Can you work these out from the drawing? Everything is in mm from the part's minimum corner. A direction names the side the tool comes from. Coordinates: 2 decimals unless noted, no trailing zeros. Order: outer loops, then holes, each group sorted by start corner. A loop starts at its lowest first (then second) coordinate and runs counter-clockwise, first axis right, second up. Notation, with made-up numbers: (-12.75, 6.5) -> (19.25, 6.5) arc R33 cw to (19.25, 41.5) -> close; hole circle Ø2 at (-36.75, -35). An arc over 180 degrees is marked (long way). Write item = value, one per line. Start each with the question number.
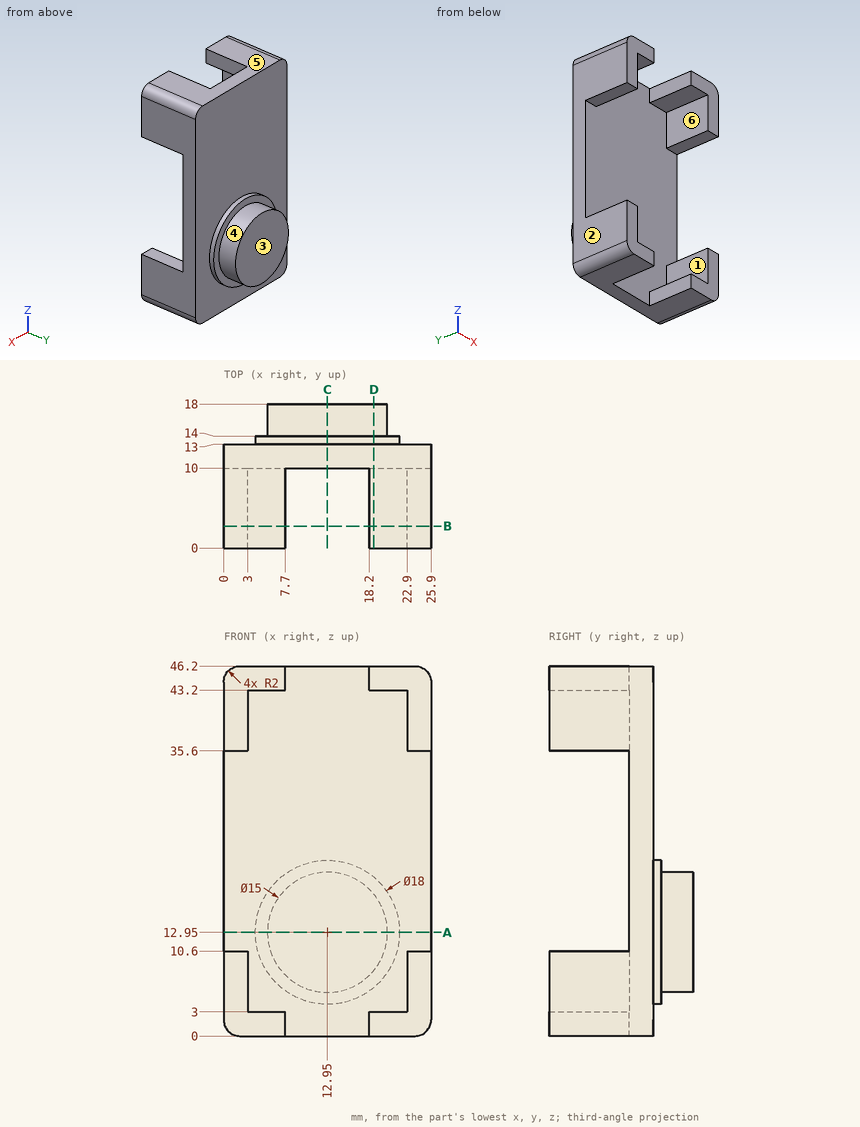
(1) Imagine slicing it at C-C (x = 12.95). Write out the boundary of the cut face in (y, z).
(2) Imagine slicing it at B-B (y = 2.75). Write out the boundary of the cut face in (x, z), plus the area to 3 significant figures.
(3) Thinking about a two-plate mould opening in Z: for the marked faces 3, 4, 5 and 6, which applies, +Z half, -Z half, draft (parallel to the pull), parting line (faces both ways), or undercut?
(4) Imagine slicing it at D-D (x = 18.75). Write out the boundary of the cut face in (y, z) (3 decimals), plus the area to 3 significant figures.
(5) Imagine slicing it at A-A (z = 12.95). Write out the boundary of the cut face in (x, y).
(6) For P1, Ø1.5, axis at x = 13.5, z = 20, coming from the -Y side, with a flat end and sliding along its axis, tell me the tip position at first contact or that it passes through.
(7) If I drill on L1, parallel to Z at x = 22.75, y = 1.5; L2, parallel to X at y = 2.25, z = 37; L3, parallel to X at y = 3.25, z = 2.5, over which ranges is the centre line in solid material (lowest first)? Write a range as from..to.
(8) For the marked faces 1 and 2, which set-ups out of +Z, -Z, +X, -X, +Y, -Y let a thin tool reach every point of the face, with its end or its side?
Result set:
q1.outline = (10, 0) -> (13, 0) -> (13, 3.95) -> (14, 3.95) -> (14, 5.45) -> (18, 5.45) -> (18, 20.45) -> (14, 20.45) -> (14, 21.95) -> (13, 21.95) -> (13, 46.2) -> (10, 46.2) -> close
q2.outline = (0, 2) arc R2 ccw to (2, 0) -> (7.7, 0) -> (7.7, 3) -> (3, 3) -> (3, 10.6) -> (0, 10.6) -> close; (0, 35.6) -> (3, 35.6) -> (3, 43.2) -> (7.7, 43.2) -> (7.7, 46.2) -> (2, 46.2) arc R2 ccw to (0, 44.2) -> close; (18.2, 0) -> (23.9, 0) arc R2 ccw to (25.9, 2) -> (25.9, 10.6) -> (22.9, 10.6) -> (22.9, 3) -> (18.2, 3) -> close; (18.2, 43.2) -> (22.9, 43.2) -> (22.9, 35.6) -> (25.9, 35.6) -> (25.9, 44.2) arc R2 ccw to (23.9, 46.2) -> (18.2, 46.2) -> close
q2.area = 180 mm2
q3.face_3 = draft
q3.face_4 = parting line
q3.face_5 = +Z half
q3.face_6 = undercut
q4.outline = (0, 0) -> (13, 0) -> (13, 6.068) -> (14, 6.068) -> (14, 8.195) -> (18, 8.195) -> (18, 17.705) -> (14, 17.705) -> (14, 19.832) -> (13, 19.832) -> (13, 46.2) -> (0, 46.2) -> (0, 43.2) -> (10, 43.2) -> (10, 3) -> (0, 3) -> close
q4.area = 250 mm2
q5.outline = (0, 10) -> (25.9, 10) -> (25.9, 13) -> (21.95, 13) -> (21.95, 14) -> (20.45, 14) -> (20.45, 18) -> (5.45, 18) -> (5.45, 14) -> (3.95, 14) -> (3.95, 13) -> (0, 13) -> close
q6.P1 = 10
q7.L1 = 0..3, 43.2..46.2
q7.L2 = 0..3, 22.9..25.9
q7.L3 = 0..7.7, 18.2..25.9
q8.face_1 = -Y
q8.face_2 = +Z, -Z, -X, +Y, -Y
